from build123d import *

# Parameters (mm, degrees)
F0_W      = 101.6
F0_H      = 101.6
F1_DEPTH  = 101.6
F2_W      = 101.6
F2_H      = 50.8
F3_DEPTH  = 76.2
F4_DEPTH  = 76.2
F5_W      = 50.8
F5_H      = 50.8
F6_DEPTH  = 25.4
F8_DEPTH  = 25.4
F10_DEPTH = 25.4
F11_W     = 50.8
F11_H     = 25.4
F12_DEPTH = 25.4


with BuildPart() as f1:
    # F0 (on Front) → F1 (new body)
    with BuildSketch(Plane.XZ):
        with Locations((-102.8639332771, -35.4373262644)):
            Rectangle(F0_W, F0_H)
    extrude(amount=F1_DEPTH)

    # F2 (on face) → F3 (cut)
    with BuildSketch(Plane.XZ.offset(101.6)):
        with Locations((-102.8639332771, -35.4373262644)):
            Rectangle(F2_W, F2_H)
    extrude(amount=-F3_DEPTH, mode=Mode.SUBTRACT)

    # F4 (cut): a face of the model
    f4_faces = [f1.faces().sort_by_distance(p)[0] for p in [
        (-102.8639332771, -101.6, 2.6626737356),
    ]]
    extrude(f4_faces, amount=-F4_DEPTH, mode=Mode.SUBTRACT)

    # F5 (on face) → F6 (cut)
    with BuildSketch(Plane.XZ.offset(25.4)):
        with Locations((-102.8639332771, -10.0373262644)):
            Rectangle(F5_W, F5_H)
    extrude(amount=-F6_DEPTH, mode=Mode.SUBTRACT)

    # F7 (on face) → F8 (cut)
    with BuildSketch(Plane.XZ.offset(25.4)):
        Polygon((-128.2639332771, 15.3626737356), (-153.6639332771, 15.3626737356), (-153.6639332771, -10.0373262644), align=None)
    extrude(amount=-F8_DEPTH, mode=Mode.SUBTRACT)

    # F9 (on face) → F10 (cut)
    with BuildSketch(Plane.XZ.offset(25.4)):
        Polygon((-52.0639332771, -10.0373262644), (-52.0639332771, 15.3626737356), (-77.4639332771, 15.3626737356), align=None)
    extrude(amount=-F10_DEPTH, mode=Mode.SUBTRACT)

    # F11 (on face) → F12 (cut)
    with BuildSketch(Plane.XY.offset(-60.8373262644)):
        with Locations((-102.8639332771, -88.9)):
            Rectangle(F11_W, F11_H)
    extrude(amount=-F12_DEPTH, mode=Mode.SUBTRACT)


solid = f1.part
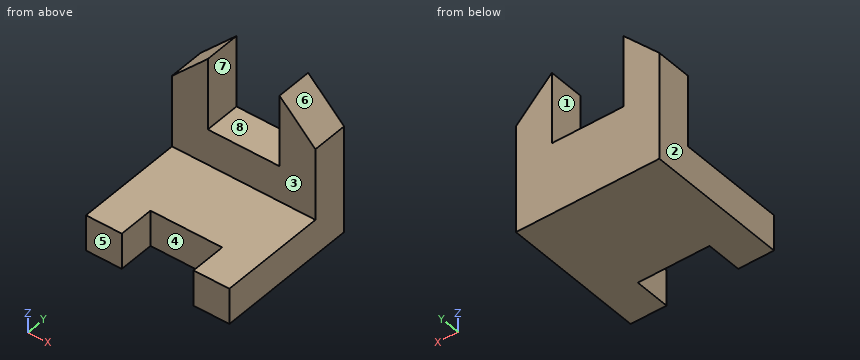
Read the model definition and answer for the solid it produces. Units are mm, in the model's axes. Face numbers are marked on the shaded views. A direction names the side the tool comes from. Coordinates: 2 decimals unless noted, no trailing zeros. Loops run counter-clockwise (first coordinate to the right, second up) from the corner with the lowest first, then second, coordinate; pieces in that order, holes last.
Q1. Consider probe 1 along X at (y, z) = (-11, -23.5); probe 2 along Y at (x, z) = (-132.5, -55.5); probe 3 along Z at (x, y) = (-72.5, -55). Determine where each line is inside the solid, lowest interval first.
Q2. The part is cut by section B-B on y = -85. Write down the section's boundary in (x, z), and give its area (3 significant figures).
Q3. The part is cut by section C-C on y = -22. Write down the section's boundary in (x, z).
Q4. The part is cut by section A-A on z = -24. Write down the section's boundary in (x, y), and give its area (3 significant figures).
Q5. Each of these flat-tipped pins is pushed along its axis until it touches: pin 1 Ø23 at (x, z) = (-91.5, -22) entering from -Y; pin 2 Ø12.5 at (x, y) = (-104.5, -15) entering from +Z; pin 3 Ø20.5 at (x, z) = (-97.5, -69) entering from -Y; pin 4 Ø3 at (x, y) = (-75, -12) entering from +Z. Where does it stop, or does it pass through?
Q6. The mould has two halves that part along X. Classify the marked faces 5, 6, 7 and 8: +X half, -X half, draft (parallel to the pull), parting line (faces both ways), or undercut.
Q7. The part is cut by section D-D on x = -112. Write down the section's boundary in (y, z).
Q8. Which of the six approach directions +Z, -Z, +X, -X, +Y, -Y give full straight-line access (tool end or side, diameter ignored) to the marked faces 1, 2, 3 and 4?
Results below:
1. probe 1: x = -153.66 to -128.26, -77.46 to -52.06
1. probe 2: y = -25.4 to 0
1. probe 3: z = -86.24 to -60.84
2. outline: (-153.66, -86.24) - (-128.26, -86.24) - (-128.26, -60.84) - (-153.66, -60.84) - close; (-77.46, -86.24) - (-52.06, -86.24) - (-52.06, -60.84) - (-77.46, -60.84) - close
2. area: 1,290 mm2
3. outline: (-153.66, -86.24) - (-52.06, -86.24) - (-52.06, -10.04) - (-77.46, 15.36) - (-77.46, -35.44) - (-128.26, -35.44) - (-128.26, 15.36) - (-153.66, -10.04) - close
4. outline: (-153.66, -25.4) - (-128.26, -25.4) - (-128.26, 0) - (-153.66, 0) - close; (-77.46, -25.4) - (-52.06, -25.4) - (-52.06, 0) - (-77.46, 0) - close
4. area: 1,290 mm2
5. pin 1: passes through
5. pin 2: stops at z = -35.44
5. pin 3: stops at y = -76.2
5. pin 4: stops at z = 14.4
6. face 5: draft
6. face 6: +X half
6. face 7: undercut
6. face 8: undercut
7. outline: (-76.2, -86.24) - (0, -86.24) - (0, -35.44) - (-25.4, -35.44) - (-25.4, -60.84) - (-76.2, -60.84) - close
8. face 1: +Z, +Y, -Y
8. face 2: +Z, -Z, -X, +Y, -Y
8. face 3: +Z, +X, -X, -Y
8. face 4: +Z, -Z, -Y
